from build123d import *

# Parameters (mm, degrees)
BOSS_EXTRUDE1_DEPTH = 5
SKETCH2_R           = 1
CUT_EXTRUDE1_DEPTH  = 5
FILLET1_R           = 1


with BuildPart() as part:
    # Sketch1 → Boss-Extrude1 (new body)
    with BuildSketch(Plane.XY):
        with BuildLine():
            Line((0, 0), (0, 3))
            Line((0, 3), (-1, 3))
            ThreePointArc((-1, 3), (-5, 7), (-9, 3))
            Line((-9, 3), (-10, 3))
            Line((-10, 3), (-10, 0))
            Line((-10, 0), (0, 0))
        make_face()
        with BuildLine():
            ThreePointArc((-7, 3), (-5, 5), (-3, 3))
            Line((-3, 3), (-7, 3))
        make_face(mode=Mode.SUBTRACT)
    extrude(amount=BOSS_EXTRUDE1_DEPTH)

    # Sketch2 → Cut-Extrude1 (cut)
    with BuildSketch(Plane.XY.offset(5)):
        with Locations((-5, 7)):
            Circle(SKETCH2_R)
        with Locations((-2.171572875, 5.828427125)):
            Circle(SKETCH2_R)
        with Locations((-7.828427125, 5.828427125)):
            Circle(SKETCH2_R)
    extrude(amount=-CUT_EXTRUDE1_DEPTH, mode=Mode.SUBTRACT)

    # Fillet1
    fillet1_edges = [part.edges().sort_by_distance(p)[0] for p in [
        (0, 3, 2.5),
        (-10, 3, 2.5),
    ]]
    fillet(fillet1_edges, radius=FILLET1_R - 0.0001)  # a hair under: the kernel refuses the full size


solid = part.part
Verification items for the finished model (mm, model axes). A direction names the side the tool comes from. Coordinates: 2 decimals unless noted, no trailing zeros. Order: outer loops, then holes, each group sorted by start corner. A loop starts at its lowest first (then second) coordinate and runs counter-clockwise, first axis right, second up.
Item 1: Depth check by flat-ended pin: pin 1 (1 mm diameter, centred on x = -8, z = 1.5, fed in from +Y). Enter the tip coordinate at first touch or a pass-through.
Filled in:
pin 1: stops at y = 5.04
Item 2: Section check A-A, the plane y = 4. Enter the section's corners in (x, z), then the cut area to 3 significant figures.
Filled in:
outline: (-8.87, 0) - (-6.73, 0) - (-6.73, 5) - (-8.87, 5) - close; (-3.27, 0) - (-1.13, 0) - (-1.13, 5) - (-3.27, 5) - close
area: 21.4 mm2
Item 3: Release check for a two-part mould opening along Y. For faces 3 (the face through (-5, 5, 2)), 4 (the face through (-5.1, 2.7, 5)), 5 (the face through (-5, 0, 2)), 6 (the face through (-5, 6, 3)) record: +Y half, -Y half, draft (parallel to the pull), parting line (faces both ways), or undercut.
Filled in:
face 3: undercut
face 4: draft
face 5: -Y half
face 6: +Y half
Item 4: Section check B-B, the plane x = -5. Enter the section's corners in (y, z), then the cut area to 3 significant figures.
Filled in:
outline: (0, 0) - (3, 0) - (3, 5) - (0, 5) - close; (5, 0) - (6, 0) - (6, 5) - (5, 5) - close
area: 20.0 mm2
Item 5: Section check D-D, the plane x = -2.5. Enter the section's corners in (y, z).
Filled in:
outline: (0, 0) - (4.88, 0) - (4.88, 5) - (0, 5) - close
Item 6: Access from +Z, -Z, +X, -X, +Y, -Y to the whole of each face (thin tool, end or side, straight path). Record for faces 1 (the face through (-5, 3, 2)), 2 (the face through (-0.285, 2.699, 2.535)).
Filled in:
face 1: +Z, -Z
face 2: +Z, -Z, +X, +Y
Item 7: Material ranges on L1, parallel to X at y = 4.25, z = 4.4; L2, parallel to X at y = 3.5, z = 3.65; L3, parallel to Y at x = -4.75, z = 0.95, recorded low to high.
Filled in:
L1: x = -8.8 to -6.56, -3.44 to -1.2
L2: x = -8.97 to -6.94, -3.06 to -1.03
L3: y = 0 to 3, 4.98 to 6.03
